```python
from build123d import *

# Parameters (mm, degrees)
F1_DEPTH = 4


with BuildPart() as f1:
    # F0 (on Front) → F1 (new body)
    with BuildSketch(Plane.XZ):
        with BuildLine():
            ThreePointArc((0, 30), (-21.213203, -21.213203), (30, 0))
            ThreePointArc((30, 0), (21.213203, 21.213203), (0, 30))
        make_face()
        with BuildLine():
            ThreePointArc((3.305106, -24.57), (-2.337063, -26.907063), (0, -21.264894))
            ThreePointArc((0, -21.264894), (2.337063, -22.232937), (3.305106, -24.57))
        make_face(mode=Mode.SUBTRACT)
        with BuildLine():
            ThreePointArc((0, -19.15), (-19.15, 0), (0, 19.15))
            ThreePointArc((0, 19.15), (13.541095, 13.541095), (19.15, 0))
            ThreePointArc((19.15, 0), (13.541095, -13.541095), (0, -19.15))
        make_face(mode=Mode.SUBTRACT)
        with BuildLine():
            ThreePointArc((0, 20.799246), (-3.775754, 24.575), (0, 28.350754))
            ThreePointArc((0, 28.350754), (2.669861, 27.244861), (3.775754, 24.575))
            ThreePointArc((3.775754, 24.575), (2.669861, 21.905139), (0, 20.799246))
        make_face(mode=Mode.SUBTRACT)
    extrude(amount=F1_DEPTH)


solid = f1.part
```
Design review of the part built by this model. Coordinates are the model's own, in mm. Round coordinates to 2 decimals unless told otherwise and drop trailing zeros. Order: outer loops, then holes, each group sorted by start corner. A loop starts at its lowest first (then second) coordinate and runs counter-clockwise, first axis right, second up. Notation, with made-up numbers: (61, 84) - (74, 84) arc R28 cw to (74, 102) - close; hole circle Ø1 at (78, 17). An arc over 180 degrees is marked (long way). One line per question, with ' | ' between items.
Item 1: Take a section at C-C, the plane z = 7. Write out the cut boundary in (x, y).
Checks:
outline: (-29.17, -4) - (-17.82, -4) - (-17.82, 0) - (-29.17, 0) - close; (17.82, -4) - (29.17, -4) - (29.17, 0) - (17.82, 0) - close
Item 2: Take a section at A-A, the plane y = -1.35. Give the number of separate pieces and of enclosed holes in the cut face, then the cut area to 3 significant figures.
Checks:
separate pieces: 1 | enclosed holes: 3 | area: 1,600 mm²
Item 3: Take a section at B-B, the plane x = -15. Write out the cut boundary in (y, z), then the cut area to 3 significant figures.
Checks:
outline: (-4, -25.98) - (0, -25.98) - (0, -11.9) - (-4, -11.9) - close; (-4, 11.9) - (0, 11.9) - (0, 25.98) - (-4, 25.98) - close | area: 113 mm²
Item 4: For P1, Ø1.5, axis at y = -1, z = 22, coming from the -X side; P2, Ø10.5, axis at x = 0, z = -24.57, coming from the -Y side; P3, Ø1, axis at x = 2, y = -1, coming from the -Z side; P4, Ø1, axis at y = -1.5, z = 18.5, coming from the -X side, all flat-tipped, find the tip position at first contact; note any pin that passes through.
Checks:
P1: x = -21.18 | P2: y = -4 | P3: z = -29.96 | P4: x = -24
Item 5: Wall thickness on line 1 (Z direction, x = 2, y = -3.3); line 2 (X direction, y = -2.9, z = -24.57); line 3 (X direction, y = -2.35, z = 10.5): over which ranges is each line inside the solid? List them lowest first. Write a range as [from, to].
Checks:
line 1: [-29.93, -27.2], [-21.94, -19.05], [19.05, 21.37], [27.78, 29.93] | line 2: [-17.21, -3.31], [3.31, 17.21] | line 3: [-28.1, -16.01], [16.01, 28.1]
